```python
from build123d import *

# Parameters (mm, degrees)
F0_R     = 9.7732259702
F0_W     = 12.7
F0_H     = 76.2
F1_DEPTH = 20.32
F2_DEPTH = 10.16
F3_R     = 7.62
F5_D     = 13.335
F6_SIZE  = 2.032
F7_DEPTH = 8.89
F9_D     = 6.35


with BuildPart() as f1:
    # F0 (on Top) → F1 (new body)
    with BuildSketch(Plane.XY):
        Polygon((-6.7755430937, 63.4059129299), (0, 63.4059129299), (12.7, 63.4059129299), (18.6244569063, 63.4059129299), (18.6244569063, 88.8059129299), (-6.7755430937, 88.8059129299), align=None)
        with Locations((6.35, 76.2461349368)):
            Circle(F0_R, mode=Mode.SUBTRACT)
        with Locations((6.35, 25.3059129299)):
            Rectangle(F0_W, F0_H)
    extrude(amount=F1_DEPTH)

    # F0 (on Top) → F2 (join)
    with BuildSketch(Plane.XY):
        with Locations((6.35, 76.2461349368)):
            Circle(F0_R)
    extrude(amount=F2_DEPTH)

    # F3
    f3_edges = [f1.edges().sort_by_distance(p)[0] for p in [
        (-3.423226, 76.246135, 10.16),
    ]]
    fillet(f3_edges, radius=F3_R)

    # F5 (through all)
    with Locations(Plane(origin=(0, 0, 0), x_dir=(0, -1, 0), z_dir=(-1, 0, 0))):
        with Locations((0.0940870701, 9.525)):
            Hole(F5_D / 2)

    # F6
    f6_edges = [f1.edges().sort_by_distance(p)[0] for p in [
        (-6.775543, 76.105913, 20.32),
        (18.624457, 76.105913, 20.32),
        (-3.387772, 63.405913, 20.32),
        (15.662228, 63.405913, 20.32),
        (5.924457, 88.805913, 20.32),
    ]]
    chamfer(f6_edges, length=F6_SIZE)

    # F0 (on Top) → F7 (join)
    with BuildSketch(Plane.XY):
        with Locations((6.35, 76.2461349368)):
            Circle(F0_R)
    extrude(amount=-F7_DEPTH)

    # F9 (through all)
    with Locations(Plane.YZ.offset(18.6244569063)):
        with Locations((76.1059129299, -4.445)):
            Hole(F9_D / 2)


solid = f1.part
```
CAD build for the part. Positions are in the model's coordinates, mm. A direction names the side the tool comes from. Coordinates: 2 decimals unless noted, no trailing zeros. Loops run counter-clockwise (first coordinate to the right, second up) from the corner with the lowest first, then second, coordinate; pieces in that order, holes last. Notation, with made-up numbers: (-22, -2) - (5, -2) arc R9 cw to (5, 4) - close; hole circle Ø7 at (14, 50). An arc over 180 degrees is marked (long way). Return JSON: item names as keys, results as strings.
1. Drop flat-ended pins along their axis: pin 1 (3 mm diameter, centred on x = 13, z = -4.5, fed in from -Y); pin 2 (16.5 mm diameter, centred on y = 7.5, z = 10.5, fed in from -X); pin 3 (7.5 mm diameter, centred on x = 10.5, y = 60.5, fed in from -Z). Give the stop position or say it passes through.
Result:
{"pin 1": "stops at y = 67.94", "pin 2": "stops at x = 0", "pin 3": "stops at z = 0"}
2. Mould opens along Z. For faces 1 (the flat face through (16, 63.406, 9)), 2 (the flat face through (-2.68, 64.41, 19.29)), 3 (the cylindrical face through (6.439, -1.539, 3.016)) say: released by +Z, released by -Z, zero draft, split by the parting line, or undercut.
Result:
{"face 1": "zero draft", "face 2": "released by +Z", "face 3": "undercut"}
3. Probe L1, parallel to Y at x = 6.5, z = 17.25; L2, parallel to Y at x = 12.5, z = 14; L3, parallel to Y at x = 2.5, z = 15. List the from-to ranges inside material, lowest first. Write a range as from..to.
Result:
{"L1": "y = -12.79..66.49, 86..88.81", "L2": "y = -12.79..-5.04, 4.85..69.99, 82.5..88.81", "L3": "y = -12.79..-3.9, 3.71..67.84, 84.65..88.81"}
4. Band-saw the part on A-A (y = -4). Give the cut face in (x, z), and give its area (3 significant figures).
Result:
{"outline": "(0, 0) - (12.7, 0) - (12.7, 4.12) - (0, 4.12) - close; (0, 14.93) - (12.7, 14.93) - (12.7, 20.32) - (0, 20.32) - close", "area": "121 mm2"}
5. Band-saw the part on C-C (z = 12). State how many separate pieces and enclosed holes the cut face has, and give its area (3 significant figures).
Result:
{"separate pieces": "2", "enclosed holes": "1", "area": "1,300 mm2"}
6. Band-saw the part on B-B (z = 1). Give the cut face in (x, y).
Result:
{"outline": "(-6.78, 63.41) - (0, 63.41) - (0, -12.79) - (12.7, -12.79) - (12.7, 63.41) - (18.62, 63.41) - (18.62, 88.81) - (-6.78, 88.81) - close"}
7. 3-axis set-ups, long thin cutter, end or side, ignore diameter. For faces 4 (the cylindrical face through (5.078, 85.936, 19.032)), 5 (the flat face through (-3, 63.406, 9)), 6 (the cylindrical face through (15.378, 72.503, -4.383)): which of +Z, -Z, +X, -X, +Y, -Y reach the whole face in a straight line?
Result:
{"face 4": "+Z", "face 5": "+Z, -Z, -X, -Y", "face 6": "-Z"}
8. Band-saw the part on D-D (y = 52). Give the cut face in (x, z), and give its area (3 significant figures).
Result:
{"outline": "(0, 0) - (12.7, 0) - (12.7, 20.32) - (0, 20.32) - close", "area": "258 mm2"}
